```python
from build123d import *

# Parameters (mm, degrees)
CYLINDER140_R           = 1.5
CYLINDER140_DEPTH       = 8
CYLINDER138_R           = 0.4
CYLINDER138_DEPTH       = 8
CYLINDER138_PITCH_ANGLE = 90
CYLINDER139_R           = 0.4
CYLINDER139_DEPTH       = 10
CYLINDER139_PITCH_ANGLE = 90
CYLINDER136_R           = 0.2
CYLINDER136_DEPTH       = 9
CYLINDER141_R           = 1.5
CYLINDER141_DEPTH       = 8
BOX028_W                = 5
BOX028_H                = 6
BOX028_DEPTH            = 1.5
BOX027_W                = 5
BOX027_H                = 6
BOX027_DEPTH            = 1.5
BOX026_W                = 5
BOX026_H                = 1.5
BOX026_DEPTH            = 1.5


with BuildPart() as bowtiemount003:
    # Cylinder140 → Cylinder140 (new body)
    with BuildSketch(Plane(origin=(127, 146.25, 63), x_dir=(1, 0, 0), z_dir=(0, 0, 1))):
        Circle(CYLINDER140_R)
    extrude(amount=CYLINDER140_DEPTH)


with BuildPart() as bowtieinjectorwire1:
    # Cylinder138 → Cylinder138 (new body)
    with BuildSketch(Plane.XY):
        Circle(CYLINDER138_R)
    extrude(amount=CYLINDER138_DEPTH)


with BuildPart() as bowtieinjectorwire1_1:
    # Cylinder138 pitch: moved
    add(bowtieinjectorwire1.part.rotate(Axis((0, 0, 0), (0, 1, 0)), CYLINDER138_PITCH_ANGLE))


with BuildPart() as bowtieinjectorwire1_2:
    # Cylinder138 placement: moved
    add(bowtieinjectorwire1_1.part.moved(Location((121.75, 148.5, 69.75))))


with BuildPart() as bowtieinjectorwire002:
    # Cylinder139 → Cylinder139 (new body)
    with BuildSketch(Plane.XY):
        Circle(CYLINDER139_R)
    extrude(amount=CYLINDER139_DEPTH)


with BuildPart() as bowtieinjectorwire002_1:
    # Cylinder139 pitch: moved
    add(bowtieinjectorwire002.part.rotate(Axis((0, 0, 0), (0, 1, 0)), CYLINDER139_PITCH_ANGLE))


with BuildPart() as bowtieinjectorwire002_2:
    # Cylinder139 placement: moved
    add(bowtieinjectorwire002_1.part.moved(Location((111, 148.5, 69.75))))


with BuildPart() as bowtienozzle004:
    # Cylinder136 → Cylinder136 (new body)
    with BuildSketch(Plane(origin=(122, 148.5, 69.5), x_dir=(1, 0, 0), z_dir=(0, 0, 1))):
        Circle(CYLINDER136_R)
    extrude(amount=CYLINDER136_DEPTH)


with BuildPart() as bowtiecut:
    # Cylinder141 → Cylinder141 (new body)
    with BuildSketch(Plane(origin=(117, 146.25, 63), x_dir=(1, 0, 0), z_dir=(0, 0, 1))):
        Circle(CYLINDER141_R)
    extrude(amount=CYLINDER141_DEPTH)

    # Fusion055: union BowTieMount003, BowTieInjectorWire1, BowTieInjectorWire002, BowTieNozzle004
    add(bowtiemount003.part)
    add(bowtieinjectorwire1_2.part)
    add(bowtieinjectorwire002_2.part)
    add(bowtienozzle004.part)


with BuildPart() as cone001:
    # Cone001 → Cone001 (revolve)
    with BuildSketch(Plane(origin=(122, 148.5, 70), x_dir=(1, 0, 0), z_dir=(0, -1, 0))):
        Polygon((0, 0), (0.7, 0), (0.5, 4), (0, 4), align=None)
    revolve(axis=Axis((122, 148.5, 70), (0, 0, 1)))


with BuildPart() as cube011:
    # Box028 → Box028 (new body)
    with BuildSketch(Plane(origin=(114.5, 143.75, 69), x_dir=(1, 0, 0), z_dir=(0, 0, 1))):
        with Locations((2.5, 3)):
            Rectangle(BOX028_W, BOX028_H)
    extrude(amount=BOX028_DEPTH)


with BuildPart() as cube010:
    # Box027 → Box027 (new body)
    with BuildSketch(Plane(origin=(124.5, 143.75, 69), x_dir=(1, 0, 0), z_dir=(0, 0, 1))):
        with Locations((2.5, 3)):
            Rectangle(BOX027_W, BOX027_H)
    extrude(amount=BOX027_DEPTH)


with BuildPart() as bowtie:
    # Box026 → Box026 (new body)
    with BuildSketch(Plane(origin=(119.5, 147.75, 69), x_dir=(1, 0, 0), z_dir=(0, 0, 1))):
        with Locations((2.5, 0.75)):
            Rectangle(BOX026_W, BOX026_H)
    extrude(amount=BOX026_DEPTH)

    # Fusion056: union Cone001, Cube011, Cube010
    add(cone001.part)
    add(cube011.part)
    add(cube010.part)

    # Cut018: cut BowTieCut
    add(bowtiecut.part, mode=Mode.SUBTRACT)


with BuildPart() as bowtie_1:
    # Cut018 placement: moved
    add(bowtie.part.moved(Location((-16.58, -0.5, -5))))


solid = bowtie_1.part
```
Here's how the part is built. I have some questions about the finished solid (model axes, mm). A direction names the side the tool comes from. Coordinates: 2 decimals unless noted, no trailing zeros. Order: outer loops, then holes, each group sorted by start corner. A loop starts at its lowest first (then second) coordinate and runs counter-clockwise, first axis right, second up. Notation, with made-up numbers: (5.5, 9) -> (33.5, 9) arc R32 cw to (33.5, 46) -> close; hole circle Ø3 at (-27, -26.75). An arc over 180 degrees is marked (long way). Return JSON: item names as keys, results as strings.
1) On a 3-axis mill with a long thin cutter (end or side, diameter ignored), from which of +Z, -Z, +X, -X, +Y, -Y can I reach the whole of each face in a straight line? I mean faces 4 (the cylindrical face through (101.124, 147.645, 64.565)), 5 (the cylindrical face through (101.226, 147.015, 64.739)), 6 (the flat face through (105, 148.75, 65)), 7 (the flat face through (105, 147.25, 65)), 8 (the flat face through (105.17, 148, 65)). Say none if no direction works.
Conclusion:
{"face 4": "-X", "face 5": "+Z, -Z", "face 6": "+Z, -Z, +Y", "face 7": "+Z, -Z, -Y", "face 8": "+X"}
2) If I drill on probe 1 along X at (y, z) = (145.75, 64.6); probe 2 along X at (y, z) = (144.05, 65.15); probe 3 along Z at (x, y) = (109.75, 148), over which ranges is the centre line in solid material (lowest first)?
Conclusion:
{"probe 1": "x = 97.92 to 98.92, 101.92 to 102.92, 107.92 to 108.92, 111.92 to 112.92", "probe 2": "x = 97.92 to 102.92, 107.92 to 112.92", "probe 3": "z = 64 to 64.35, 65.15 to 65.5"}
3) If we section it at A-A on x = 100.42: List the corners of the cut face in (y, z) for me.
Conclusion:
{"outline": "(143.25, 64) -> (144.25, 64) -> (144.25, 65.5) -> (143.25, 65.5) -> close; (147.25, 64) -> (149.25, 64) -> (149.25, 65.5) -> (147.25, 65.5) -> close; hole circle Ø0.8 at (148, 64.75)"}
4) Thinking about a two-plate mould opening in Z: for faces 1 (the flat face through (104.42, 148, 65)), 2 (the flat face through (110, 143.25, 65)), 3 (the conical face through (105.962, 147.775, 67.274)), which applies, +Z half, -Z half, draft (parallel to the pull), parting line (faces both ways), or undercut?
Conclusion:
{"face 1": "undercut", "face 2": "draft", "face 3": "+Z half"}
5) I'm going to push flat-ended pins straight in: P1, Ø2, axis at x = 106.5, z = 67.5, coming from the -Y side; P2, Ø1, axis at x = 102.5, y = 147, coming from the +Z side; P3, Ø1.2, axis at x = 105.5, z = 64.5, coming from the -Y side. Where does each tip first touch, or does it pass through?
Conclusion:
{"P1": "stops at y = 147.42", "P2": "stops at z = 65.5", "P3": "stops at y = 147.25"}
6) If we section it at C-C on x = 105.42: List the corners of the cut face in (y, z) for me (3 decimals), plus the area to 3 significant figures.
Conclusion:
{"outline": "(147.25, 64) -> (148.75, 64) -> (148.75, 65.5) -> (148.675, 65.5) -> (148.5, 69) -> (148.2, 69) -> (148.2, 65.096) arc R0.4 cw (long way) to (147.8, 65.096) -> (147.8, 69) -> (147.5, 69) -> (147.325, 65.5) -> (147.25, 65.5) -> close", "area": "4.31 mm²"}
7) If we section it at B-B on y = 143.9: List the corners of the cut face in (x, z) for me.
Conclusion:
{"outline": "(97.92, 64) -> (102.92, 64) -> (102.92, 65.5) -> (97.92, 65.5) -> close; (107.92, 64) -> (112.92, 64) -> (112.92, 65.5) -> (107.92, 65.5) -> close"}
8) If we section it at D-D on z = 64.75: List the corners of the cut face in (x, y) for me.
Conclusion:
{"outline": "(97.92, 143.25) -> (102.92, 143.25) -> (102.92, 147.25) -> (107.92, 147.25) -> (107.92, 143.25) -> (112.92, 143.25) -> (112.92, 147.6) -> (105.17, 147.6) -> (105.17, 148.4) -> (112.92, 148.4) -> (112.92, 149.25) -> (107.92, 149.25) -> (107.92, 148.75) -> (102.92, 148.75) -> (102.92, 149.25) -> (97.92, 149.25) -> (97.92, 148.4) -> (104.42, 148.4) -> (104.42, 147.6) -> (97.92, 147.6) -> close; hole circle Ø3 at (100.42, 145.75); hole circle Ø3 at (110.42, 145.75)"}
